```python
from build123d import *

# Parameters (mm, degrees)
SKETCH1_W           = 52.5
SKETCH1_H           = 52.5
BOSS_EXTRUDE1_DEPTH = 2
SKETCH1_3_R         = 2.85
SKETCH1_3_R_2       = 1.25
BOSS_EXTRUDE2_DEPTH = 25
FILLET1_R           = 4
FILLET2_R           = 1.2
FILLET3_R           = 2
FILLET4_R           = 4


with BuildPart() as part:
    # Sketch1 → Boss-Extrude1 (new body)
    with BuildSketch(Plane.XY):
        with Locations((-13.622062437, -11.00131333)):
            Rectangle(SKETCH1_W, SKETCH1_H)
        Polygon((-32.122062437, 4.670259545), (-16.450489562, -11.00131333), (-32.122062437, -26.672886205), align=None, mode=Mode.SUBTRACT)
        Polygon((-29.293635312, 7.49868667), (2.049510438, 7.49868667), (-13.622062437, -8.172886205), align=None, mode=Mode.SUBTRACT)
        Polygon((-29.293635312, -29.50131333), (2.049510438, -29.50131333), (-13.622062437, -13.829740455), align=None, mode=Mode.SUBTRACT)
        Polygon((4.877937563, 4.670259545), (4.877937563, -26.672886205), (-10.793635312, -11.00131333), align=None, mode=Mode.SUBTRACT)
    extrude(amount=BOSS_EXTRUDE1_DEPTH)

    # Sketch1_3 → Boss-Extrude2 (add)
    # profile 1 of 4: a face of its own
    with BuildSketch(Plane.XY):
        with Locations((-35.622062437, 10.99868667)):
            Circle(SKETCH1_3_R)
        with Locations((-35.622062437, 10.99868667)):
            Circle(SKETCH1_3_R_2, mode=Mode.SUBTRACT)
    # profile 2 of 4: a face of its own
    with BuildSketch(Plane.XY):
        with Locations((-35.622062437, -33.00131333)):
            Circle(SKETCH1_3_R)
        with Locations((-35.622062437, -33.00131333)):
            Circle(SKETCH1_3_R_2, mode=Mode.SUBTRACT)
    # profile 3 of 4: a face of its own
    with BuildSketch(Plane.XY):
        with Locations((8.377937563, -33.00131333)):
            Circle(SKETCH1_3_R)
        with Locations((8.377937563, -33.00131333)):
            Circle(SKETCH1_3_R_2, mode=Mode.SUBTRACT)
    # profile 4 of 4: a face of its own
    with BuildSketch(Plane.XY):
        with Locations((8.377937563, 10.99868667)):
            Circle(SKETCH1_3_R)
        with Locations((8.377937563, 10.99868667)):
            Circle(SKETCH1_3_R_2, mode=Mode.SUBTRACT)
    extrude(amount=-BOSS_EXTRUDE2_DEPTH)

    # Fillet1
    fillet1_edges = [part.edges().sort_by_distance(p)[0] for p in [
        (12.627937563, -37.25131333, 1),
        (-39.872062437, -37.25131333, 1),
        (-39.872062437, 15.24868667, 1),
        (12.627937563, 15.24868667, 1),
    ]]
    fillet(fillet1_edges, radius=FILLET1_R)

    # Fillet2
    fillet2_edges = [part.edges().sort_by_distance(p)[0] for p in [
        (-38.472062437, 10.99868667, 0),
        (-38.472062437, -33.00131333, 0),
        (5.527937563, -33.00131333, 0),
        (5.527937563, 10.99868667, 0),
    ]]
    fillet(fillet2_edges, radius=FILLET2_R)

    # Fillet3
    fillet3_edges = [part.edges().sort_by_distance(p)[0] for p in [
        (-29.293635312, -29.50131333, 1),
        (2.049510438, -29.50131333, 1),
        (2.049510438, 7.49868667, 1),
        (-29.293635312, 7.49868667, 1),
        (-32.122062437, 4.670259545, 1),
        (-32.122062437, -26.672886205, 1),
        (4.877937563, -26.672886205, 1),
        (4.877937563, 4.670259545, 1),
    ]]
    fillet(fillet3_edges, radius=FILLET3_R)

    # Fillet4
    fillet4_edges = [part.edges().sort_by_distance(p)[0] for p in [
        (-13.622062437, -13.829740455, 1),
        (-13.622062437, -8.172886205, 1),
        (-16.450489562, -11.00131333, 1),
        (-10.793635312, -11.00131333, 1),
    ]]
    fillet(fillet4_edges, radius=FILLET4_R)


solid = part.part
```
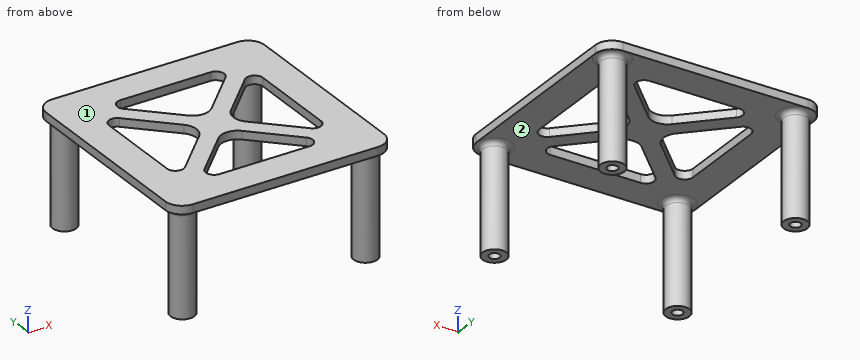
For this review, take the finished solid that the model builds, in its own axes (mm). Face numbers are marked on the shaded views. Give positions to 0.01 mm unless a question says otherwise; leave off trailing zeros. Write each loop counter-clockwise with the first axis right and the second up, starting at its lowest first coordinate (ties: lowest second). Pieces come first, ordered by that corner, then holes. Notation, with made-up numbers: M 63.25,1 L 86.25,1 A23 ccw 86.25,40 Z; hole C -25.5,24.5 d2. An arc over 180 degrees is marked long. One line per item, written item: value.
1) For line 1 (X direction, y = -33.5, z = -16.75); line 2 (Y direction, x = -36, z = -1.5); line 3 (X direction, y = -34, z = -8.25), list the stretches that pass through material, from the lowest coordinate up. Write a range as from..to.
Results are:
line 1: x = -38.43..-36.77, -34.48..-32.82, 5.57..7.23, 9.52..11.18
line 2: y = -35.83..-34.19, -31.81..-30.18, 8.17..9.81, 12.19..13.82
line 3: x = -38.29..-36.37, -34.87..-32.95, 5.71..7.63, 9.13..11.05
2) Take a section at D-D, the plane x = -5.5. Write out the cut boundary in (y, z), then the cut area to 3 significant figures.
Results are:
outline: M -37.25,0 L -29.5,0 L -29.5,2 L -37.25,2 Z; M -21.95,0 L -16.29,0 L -16.29,2 L -21.95,2 Z; M -5.71,0 L -0.05,0 L -0.05,2 L -5.71,2 Z; M 7.5,0 L 15.25,0 L 15.25,2 L 7.5,2 Z
area: 53.6 mm²
3) Take a section at B-B, the plane y = -11. Write out the cut boundary in (x, z).
Results are:
outline: M -39.87,0 L -32.12,0 L -32.12,2 L -39.87,2 Z; M -18.11,0 L -9.14,0 L -9.14,2 L -18.11,2 Z; M 4.88,0 L 12.63,0 L 12.63,2 L 4.88,2 Z
4) Take a section at A-A, the plane z = -8.5. Write out the cut boundary in (x, y), then the cut area to 3 significant figures.
Results are:
outline: C -35.62,-33 d5.7; C -35.62,11 d5.7; C 8.38,-33 d5.7; C 8.38,11 d5.7; hole C -35.62,-33 d2.5; hole C -35.62,11 d2.5; hole C 8.38,-33 d2.5; hole C 8.38,11 d2.5
area: 82.4 mm²
5) Take a section at C-C, the plane y = -22.5. Write out the cut boundary in (x, z), then the cut area to 3 significant figures.
Results are:
outline: M -39.87,0 L -32.01,0 L -32.01,2 L -39.87,2 Z; M -27.95,0 L -22.29,0 L -22.29,2 L -27.95,2 Z; M -4.95,0 L 0.71,0 L 0.71,2 L -4.95,2 Z; M 4.77,0 L 12.63,0 L 12.63,2 L 4.77,2 Z
area: 54.1 mm²
6) The part is to be moulded in two halves that separate along X. For the marked faces 1 and 2, say which applies: +X half, -X half, draft (parallel to the pull), parting line (faces both ways), or undercut.
Results are:
face 1: draft
face 2: undercut
7) For P1, Ø4, axis at y = -3.5, z = -2.5, coming from the +X side; P2, Ø5, axis at x = -33, y = 0, coming from the -Z side; P3, Ø12, axis at x = -33.5, z = -9.5, coming from the -Y side; P4, Ø10, axis at x = 4.5, z = -22, coming from the +Y side, all flat-tipped, find the tip position at first contact; note any pin that passes through.
Results are:
P1: passes through
P2: stops at z = 0
P3: stops at y = -35.85
P4: stops at y = 13.85
